Autodesk Inventor part; units mm, degrees
ref_plane "YZ Plane" through (0, 0, 0) normal (1, 0, 0) x (0, 1, 0)
ref_plane "XZ Plane" through (0, 0, 0) normal (0, 1, 0) x (-1, 0, 0)
ref_plane "XY Plane" through (0, 0, 0) normal (0, 0, 1) x (1, 0, 0)
sketch "Sketch1" plane through (0, 0, 0) normal (0, 0, 1) x (1, 0, 0)
  line L0 (0, 0) -> (160, 0)
  line L1 (160, 0) -> (160, 60)
  line L2 (160, 60) -> (0, 60)
  line L3 (0, 60) -> (0, 0)
  dimension "d0" = 160
  dimension "d1" = 60
extrude "Extrusion1" add sketch "Sketch1" along normal blind 6
sketch "Sketch2" plane through (0, 0, 0) normal (0, -1, 0) x (1, 0, 0)
  line L0 (3, 3) -> (157, 3) construction
  line L1 (160, 0) -> (0, 0) construction
  line L2 (0, 6) -> (160, 6) construction
  line L3 (160, 0) -> (160, 6) construction
  line L4 (0, 0) -> (0, 6) construction
  point P0 (0, 3)
  dimension "d4" = 3
  dimension "d5" = 6
  dimension "d6" = 3
  dimension "d7" = 3
hole "Hole1" at (3, 0, 3) at (157, 0, 3) direction (0, 1, 0) diameter 2.459 depth 8.8 tip angle 118
chamfer "Chamfer1" distance 0.3 angle 45 2 edges at (3, 0, 4.2295) (157, 0, 4.2295)
sketch "Sketch3" plane through (0, 60, 0) normal (0, 1, 0) x (1, 0, 0)
  line L0 (160, -6) -> (0, -6)
  line L1 (148, -6) -> (145, -3)
  line L2 (148, -6) -> (152.2426, -6) construction
  line L3 (145, -3) -> (15, -3)
  line L4 (160, 0) -> (0, 0)
  line L5 (15, -3) -> (12, -6)
  line L6 (12, -6) -> (148, -6)
  line L7 (160, 0) -> (160, -6)
  line L8 (0, 0) -> (0, -6)
  point P0 (12, -6)
  point P1 (0, -3)
  dimension "d18" = 135
  dimension "d19" = 3
  dimension "d22" = 15
  dimension "d23" = 130
  dimension "d24" = 15
extrude "Extrusion2" cut sketch "Sketch3" against normal through all contours L0 L5 L3 L1
sketch "Sketch6" plane through (160, 0, 0) normal (1, 0, 0) x (0, 0, -1)
  line L0 (-3, 60) -> (-3, 0)
  circle A0 centre (-3, 12.5) radius 1.5
  circle A1 centre (-3, 47.5) radius 1.5
  line L1 (0, 0) -> (-6, 0)
  line L2 (0, 60) -> (-6, 60)
  dimension "d34" = 3
  dimension "d35" = 3
  dimension "d36" = 35
  dimension "d37" = 12.5
  dimension "d38" = 60
hole "Hole2" at (160, 12.5, 3) at (160, 47.5, 3) direction (-1, 0, 0) diameter 2.459 depth 8.8 tip angle 118
sketch "Sketch7" plane through (0, 0, 0) normal (-1, 0, 0) x (0, 0, 1)
  line L0 (3, 60) -> (3, 0)
  circle A0 centre (3, 12.5) radius 1.5
  circle A1 centre (3, 47.5) radius 1.5
  line L1 (0, 60) -> (6, 60)
  line L2 (0, 0) -> (6, 0)
  dimension "d46" = 3
  dimension "d47" = 3
  dimension "d48" = 35
  dimension "d49" = 60
  dimension "d50" = 12.5
hole "Hole3" at (0, 47.5, 3) at (0, 12.5, 3) direction (1, 0, 0) diameter 2.459 depth 8.8 tip angle 118
chamfer "Chamfer2" distance 0.3 angle 45 4 edges at (0, 47.5, 1.7705) (0, 12.5, 1.7705) (160, 47.5, 4.2295) (160, 12.5, 4.2295)
equation "\"d4\" = 0.5 * d5"
equation "\"d22\" = d24"
equation "\"d37\" = -0.5 * d36 + 0.5 * d38"
equation "\"d50\" = -0.5 * d48 + 0.5 * d49"
properties part number "Prawa ściana"
CAD build for the part. Positions are in the model's coordinates, mm. A direction names the side the tool comes from. Coordinates: 2 decimals unless noted, no trailing zeros. Loops run counter-clockwise (first coordinate to the right, second up) from the corner with the lowest first, then second, coordinate; pieces in that order, holes last. Notation, with made-up numbers: (24, -23.75) - (42, -23.75) arc R22 cw to (42, 9.25) - close; hole circle Ø8 at (-2.75, -31). An arc over 180 degrees is marked (long way). Write item = value, one per line. Start each with the question number.
Q1. Cut at B-B, the plane x = 48. List the corners of the cut face in (y, z).
Q2. Drill centre lines: L1, parallel to Y at x = 155.5, z = 3; L2, parallel to Z at x = 153.5, y = 12.5; L3, parallel to X at y = 5.5, z = 2.75. Where is each one in solid material? Low to high.
Q3. Which spindle directions (+Z, -Z, +X, -X, +Y, -Y) get a long thin tool onto all of the face, cutting with end or side? Do faces 4 (the flat face through (6, 30, 6)), 5 (the flat face through (147, 30, 5)). Say none if no direction does.
Q4. Flat gauge pins, fed straight in: pin 1 Ø3 at (y, z) = (47.5, 3) entering from -X; pin 2 Ø2 at (y, z) = (47.5, 3) entering from +X; pin 3 Ø3 at (x, z) = (3, 3) entering from -Y. Where does each tip first touch, or does it go through?
Q5. Cut at A-A, the plane y = 34.5. List the corners of the cut face in (x, z), then the cut area to 3 significant figures.
Q6. Pull direction X, two halves, no side cores. Call faces 1 (the flat face through (81, 30, 3)), 2 (the flat face through (154, 30, 6)), 3 (the flat face through (0, 30, 3)): pulls with the +X half, pulls with the -X half, needs draft (parallel to the pull), parting line crosses it, or undercut.
Computed:
q1.outline = (0, 0) - (60, 0) - (60, 3) - (0, 3) - close
q2.L1 = 0.03 to 11.27, 13.73 to 46.27, 48.73 to 60
q2.L2 = 0 to 1.77, 4.23 to 6
q2.L3 = 0 to 1.8, 4.2 to 155.8, 158.2 to 160
q3.face_4 = +Z, +X, -X, +Y, -Y
q3.face_5 = +Z, +Y, -Y
q4.pin_1 = 0.03
q4.pin_2 = 151.06
q4.pin_3 = 0.03
q5.outline = (0, 0) - (160, 0) - (160, 6) - (148, 6) - (145, 3) - (15, 3) - (12, 6) - (0, 6) - close
q5.area = 561 mm²
q6.face_1 = undercut
q6.face_2 = needs draft
q6.face_3 = pulls with the -X half
